Source: CAD feature listing. Evaluate the final solid. Frame: model axes, mm. A direction names the side the tool comes from. Give positions to 0.01 mm unless a question says otherwise; leave off trailing zeros. Loops run counter-clockwise (first coordinate to the right, second up) from the corner with the lowest first, then second, coordinate; pieces in that order, holes last. Notation, with made-up numbers: (89.25, -3.75) -> (132.25, -3.75) arc R20 cw to (132.25, 17.25) -> close; hole circle Ø4 at (-39, -33). An arc over 180 degrees is marked (long way). Put each result on its own line as item: value.
```python
from build123d import *

# Parameters (mm, degrees)
SKETCH1_W                  = 11
SKETCH1_H                  = 9
BOSS_EXTRUDE1_DEPTH        = 80
BOSS_EXTRUDE2_DEPTH        = 10
F_3_9_3_9_DIAMETER_HOLE1_D = 3.9
CHAMFER1_SIZE              = 4
M6X1_0_TAPPED_HOLE1_D      = 5
M6X1_0_TAPPED_HOLE1_DEPTH  = 15
M6X1_0_TAPPED_HOLE1_TIP    = 1.502151548


with BuildPart() as part:
    # Sketch1 → Boss-Extrude1 (new body)
    with BuildSketch(Plane(origin=(0, 0, 0), x_dir=(1, 0, 0), z_dir=(0, 1, 0))):
        with Locations((0, -4.5)):
            Rectangle(SKETCH1_W, SKETCH1_H)
    extrude(amount=-BOSS_EXTRUDE1_DEPTH)

    # Sketch2 → Boss-Extrude2 (add)
    with BuildSketch(Plane(origin=(0, 0, 0), x_dir=(1, 0, 0), z_dir=(0, 1, 0))):
        Polygon((-9.5, 3), (-9.5, -4), (9.5, -4), (9.5, 3), (18, 3), (18, -9), (-18, -9), (-18, 3), align=None)
    extrude(amount=BOSS_EXTRUDE2_DEPTH)

    # Ø3.9 (3.9) Diameter Hole1 (through all)
    with Locations(Plane(origin=(0, 0, -3), x_dir=(-1, 0, 0), z_dir=(0, 0, -1))):
        with Locations((-13.25, 5), (13.25, 5)):
            Hole(F_3_9_3_9_DIAMETER_HOLE1_D / 2)

    # Chamfer1
    chamfer1_edges = [part.edges().sort_by_distance(p)[0] for p in [
        (-5.5, 0, 6.5),
        (5.5, 0, 6.5),
    ]]
    chamfer(chamfer1_edges, length=CHAMFER1_SIZE)
    chamfer1_2_edges = [part.edges().sort_by_distance(p)[0] for p in [
        (0, 0, 0),
    ]]
    chamfer(chamfer1_2_edges, length=CHAMFER1_SIZE - 0.0001)  # a hair under: the kernel refuses the full size

    # M6x1.0 Tapped Hole1
    with Locations(Plane(origin=(0, -80, 0), x_dir=(-1, 0, 0), z_dir=(0, -1, 0))):
        with Locations((0, -4.5)):
            Hole(M6X1_0_TAPPED_HOLE1_D / 2, depth=M6X1_0_TAPPED_HOLE1_DEPTH)
            with Locations((0, 0, -(M6X1_0_TAPPED_HOLE1_DEPTH + M6X1_0_TAPPED_HOLE1_TIP / 2))):  # 118° drill point
                Cone(0, M6X1_0_TAPPED_HOLE1_D / 2, M6X1_0_TAPPED_HOLE1_TIP, mode=Mode.SUBTRACT)


solid = part.part
```
(1) Section A-A on z = -1.5. Return loops of the section in (x, y).
Calculated:
outline: (-18, 0) -> (-9.5, 0) -> (-9.5, 10) -> (-18, 10) -> close; (9.5, 0) -> (18, 0) -> (18, 10) -> (9.5, 10) -> close; hole circle Ø3.9 at (-13.25, 5); hole circle Ø3.9 at (13.25, 5)
(2) Reachability of faces 4 (the flat face through (0, 4, 4)), 5 (the flat face through (-18, 5, 3)), 6 (the flat face through (-14, 0, 3)), 7 (the cylindrical face through (0, -72, 2)) from +Z, -Z, +X, -X, +Y, -Y: full face, straight path, thin tool, end or side. Return the list, or none.
Calculated:
face 4: -Z, +Y
face 5: +Z, -Z, -X, +Y, -Y
face 6: +Z, -Z, -X, -Y
face 7: -Y
(3) First-contact query: P1, Ø2, axis at x = 8, y = -32, coming from the -Z side; P2, Ø12, axis at x = 3.5, y = -62, coming from the -Z side; P3, Ø7, axis at x = -12, z = 5, coming from the -Y side; P4, Ø4, axis at x = 0, z = 4.5, coming from the -Y side. Flat tips, straight axial feed; report the tip coordinate or a pass-through.
Calculated:
P1: passes through
P2: stops at z = 0
P3: stops at y = -1
P4: stops at y = -64.7
(4) Line query: probe 1 along Y at (x, z) = (13.25, -0.5); probe 2 along Z at (x, y) = (0, -68.25); probe 3 along X at (y, z) = (-21, 1.75). Output: solid intervals per line, ascending. Write a range as from..to.
Calculated:
probe 1: y = 0..3.05, 6.95..10
probe 2: z = 0..2, 7..9
probe 3: x = -5.5..5.5
(5) Section B-B on y = 5. Return loops of the section in (x, z).
Calculated:
outline: (-18, -3) -> (-15.2, -3) -> (-15.2, 9) -> (-18, 9) -> close; (-11.3, -3) -> (-9.5, -3) -> (-9.5, 4) -> (9.5, 4) -> (9.5, -3) -> (11.3, -3) -> (11.3, 9) -> (-11.3, 9) -> close; (15.2, -3) -> (18, -3) -> (18, 9) -> (15.2, 9) -> close
(6) Section C-C on x = 13.25. Return loops of the section in (y, z), then the cut area to 3 significant figures.
Calculated:
outline: (0, -3) -> (3.05, -3) -> (3.05, 9) -> (0, 9) -> close; (6.95, -3) -> (10, -3) -> (10, 9) -> (6.95, 9) -> close
area: 73.2 mm²
(7) Section D-D on y = -72.5. Return loops of the section in (x, z), then the cut area to 3 significant figures.
Calculated:
outline: (-5.5, 0) -> (5.5, 0) -> (5.5, 9) -> (-5.5, 9) -> close; hole circle Ø5 at (0, 4.5)
area: 79.4 mm²
(8) Draft query along X for faces 1 (the flat face through (-9.5, 5, 0)), 2 (the flat face through (18, 5, 3)), 3 (the flat face through (14, 0, 3)). Return one class per face: released by +X, released by -X, zero draft, split by the parting line, or undercut.
Calculated:
face 1: undercut
face 2: released by +X
face 3: zero draft
